from build123d import *

# Parameters (mm, degrees)
F1_DEPTH = 4.5
F2_R     = 1
F4_DEPTH = 25


with BuildPart() as f1:
    # F0 (on Front) → F1 (new body)
    with BuildSketch(Plane.XZ):
        with BuildLine():
            ThreePointArc((0, 10.9), (7.707464, 7.707464), (10.9, 0))
            ThreePointArc((10.9, 0), (10.528592, -2.821128), (9.439677, -5.45))
            Line((9.439677, -5.45), (34.641016, -20))
            Line((34.641016, -20), (18.084448, -2.966725))
            Line((18.084448, -2.966725), (7.698172, 12.818934))
            Line((7.698172, 12.818934), (0, 40))
            Line((0, 40), (0, 10.9))
        make_face()
        with BuildLine():
            ThreePointArc((-9.439677, -5.45), (-9.439677, 5.45), (0, 10.9))
            Line((0, 10.9), (0, 40))
            Line((0, 40), (-7.25986, 14.366547))
            Line((-7.25986, 14.366547), (-18.265326, -3.152812))
            Line((-18.265326, -3.152812), (-34.641016, -20))
            Line((-34.641016, -20), (-9.439677, -5.45))
        make_face()
        with BuildLine():
            Line((34.641016, -20), (9.439677, -5.45))
            ThreePointArc((9.439677, -5.45), (0, -10.9), (-9.439677, -5.45))
            Line((-9.439677, -5.45), (-34.641016, -20))
            Line((-34.641016, -20), (-8.926296, -13.499424))
            Line((-8.926296, -13.499424), (8.926296, -13.499424))
            Line((8.926296, -13.499424), (34.641016, -20))
        make_face()
    extrude(amount=F1_DEPTH)

    # F2
    f2_edges = [f1.edges().sort_by_distance(p)[0] for p in [
        (0, -2.25, 40),
        (34.641016, -2.25, -20),
        (-34.641016, -2.25, -20),
    ]]
    fillet(f2_edges, radius=F2_R)

    # F3 (on face) → F4 (cut)
    with BuildSketch(Plane(origin=(0, 0, 0), x_dir=(-1, 0, 0), z_dir=(0, 1, 0))):
        Polygon((-11.210982, -11.404401), (-9.875284, -7.285431), (-12.774568, -4.069198), (-17.009549, -4.971935), (-18.345247, -9.090904), (-15.445963, -12.307137), align=None)
        Polygon((17.32114, -10.724252), (18.027603, -6.452143), (14.68108, -3.704275), (10.628094, -5.228514), (9.921631, -9.500623), (13.268154, -12.248491), align=None)
        Polygon((0.09283, 12.183193), (3.795553, 14.428152), (3.702723, 18.757284), (-0.09283, 20.841457), (-3.795553, 18.596498), (-3.702723, 14.267366), align=None)
    extrude(amount=-F4_DEPTH, mode=Mode.SUBTRACT)


solid = f1.part
Design review of the part built by this model. Coordinates are the model's own, in mm. A direction names the side the tool comes from. Give positions to 0.01 mm unless a question says otherwise; leave off trailing zeros. Order: outer loops, then holes, each group sorted by start corner. A loop starts at its lowest first (then second) coordinate and runs counter-clockwise, first axis right, second up.
1. Mouldability with a two-part tool opening along Z and no side actions: class faces 4 (the flat face through (19.92, -2.22, -16.28)), 5 (the flat face through (-25.125, -2.218, -10.21)), 6 (the flat face through (10.55, -2.22, -9.37)), 7 (the flat face through (-15.266, -2.218, -11.497)) as +Z half, -Z half, draft (parallel to the pull), parting line (faces both ways), or undercut.
Solution:
face 4: -Z half
face 5: +Z half
face 6: undercut
face 7: undercut
2. Add section D-D, the plane x = 24.5. State the section outline as (y, z) points, then the cut area to 3 significant figures.
Solution:
outline: (-4.5, -17.44) - (0, -17.44) - (0, -9.57) - (-4.5, -9.57) - close
area: 35.4 mm2
3. Add section B-B, the plane z = 1.5. State the section outline as (x, y) points, then the cut area to 3 significant figures.
Solution:
outline: (-15.34, -4.5) - (-10.8, -4.5) - (-10.8, 0) - (-15.34, 0) - close; (10.8, -4.5) - (15.15, -4.5) - (15.15, 0) - (10.8, 0) - close
area: 40.0 mm2
4. To check wall thickness, follow L1, parallel to X at y = -4.05, z = -8.5; L2, parallel to Z at x = -0.5, y = -0.55; L3, parallel to X at y = -0.5, z = -8. State the ranges of each line that lie inside material, in increasing order.
Solution:
L1: x = -23.46 to -17.69, -10.09 to -6.82, 6.82 to 10.27, 18.15 to 23.46
L2: z = -13.5 to -10.89, 10.89 to 12.43, 20.52 to 37.2
L3: x = -22.98 to -17.77, -10.17 to -7.4, 7.4 to 10.11, 17.99 to 22.98
5. Tool access review of faces 1 (the flat face through (0, -2, -13.499)), 2 (the flat face through (11.305, -2.218, -5.7)), 3 (the flat face through (12.96, -2.22, 4.82)): name each direction out of +Z, -Z, +X, -X, +Y, -Y from which nothing blocks a thin tool from reaching the whole face with its end or side.
Solution:
face 1: -Z, +Y, -Y
face 2: +Y, -Y
face 3: +Z, +X, +Y, -Y
6. Add section A-A, the plane y = -1.35. State how many separate pieces and enclosed holes the cut face has, then the cut area to 3 significant figures.
Solution:
separate pieces: 1
enclosed holes: 4
area: 710 mm2
7. Add section C-C, the plane z = 17. State the section outline as (x, y) points.
Solution:
outline: (-6.51, -4.5) - (-3.74, -4.5) - (-3.74, 0) - (-6.51, 0) - close; (3.76, -4.5) - (6.51, -4.5) - (6.51, 0) - (3.76, 0) - close
8. For pin 1 Ø1.5 at (y, z) = (-4, -13) entering from -X; pin 2 Ø3 at (x, z) = (5, 24) entering from -Y, all flat-tipped, find the tip position at first contact; note any pin that passes through.
Solution:
pin 1: stops at x = -28.57
pin 2: stops at y = -4.5
